Could you check a few things on this model? Use its own coordinates, in mm. Face numbers are marked on the shaded views. A direction names the side the tool comes from. Coordinates: 2 decimals unless noted, no trailing zeros. Loops run counter-clockwise (first coordinate to the right, second up) from the corner with the lowest first, then second, coordinate; pieces in that order, holes last. Notation, with made-up numbers: M -13,-6.75 L -8,-6.75 A22 cw -8,23.25 Z; hole C 86,26.25 d11. An arc over 180 degrees is marked long. Write each question's results on one line, items separated by ' | '.
```python
from build123d import *

# Parameters (mm, degrees)
SKETCH1_W                  = 26
SKETCH1_H                  = 24
BOSS_EXTRUDE1_DEPTH        = 12
CUT_EXTRUDE1_DEPTH         = 30.816103032
M3_CLEARANCE_HOLE1_D       = 3.242
M3_CLEARANCE_HOLE1_DEPTH   = 6.064115214
M3_CLEARANCE_HOLE1_TIP     = 0.935884786
F_4_5_4_5_DIAMETER_HOLE1_D = 4.5
CHAMFER1_SIZE              = 0.379


with BuildPart() as part:
    # Sketch1 → Boss-Extrude1 (new body)
    with BuildSketch(Plane.XY.offset(6)):
        with Locations((0, 12)):
            Rectangle(SKETCH1_W, SKETCH1_H)
    extrude(amount=-BOSS_EXTRUDE1_DEPTH)

    # Sketch2 → Cut-Extrude1 (cut, through all)
    with BuildSketch(Plane(origin=(0, 0, -6), x_dir=(-1, 0, 0), z_dir=(0, 0, -1))):
        with BuildLine():
            Line((3.01340754, 24), (-3.01340754, 24))
            ThreePointArc((-3.01340754, 24), (0, 21.825), (3.01340754, 24))
        make_face()
    extrude(amount=-CUT_EXTRUDE1_DEPTH, mode=Mode.SUBTRACT)

    # M3 Clearance Hole1
    with Locations(Plane(origin=(0, 24, 0), x_dir=(1, 0, 0), z_dir=(0, 1, 0))):
        with Locations((8, 0), (-8, 0)):
            Hole(M3_CLEARANCE_HOLE1_D / 2, depth=M3_CLEARANCE_HOLE1_DEPTH)
            with Locations((0, 0, -(M3_CLEARANCE_HOLE1_DEPTH + M3_CLEARANCE_HOLE1_TIP / 2))):  # 120° drill point
                Cone(0, M3_CLEARANCE_HOLE1_D / 2, M3_CLEARANCE_HOLE1_TIP, mode=Mode.SUBTRACT)

    # Ø4.5 (4.5) Diameter Hole1 (through all)
    with Locations(Plane.XY.offset(6)):
        with Locations((8, 5), (-8, 5)):
            Hole(F_4_5_4_5_DIAMETER_HOLE1_D / 2)

    # Chamfer1
    chamfer1_edges = [part.edges().sort_by_distance(p)[0] for p in [
        (-6.379, 24, 0),
        (9.621, 24, 0),
    ]]
    chamfer(chamfer1_edges, length=CHAMFER1_SIZE)


solid = part.part
```
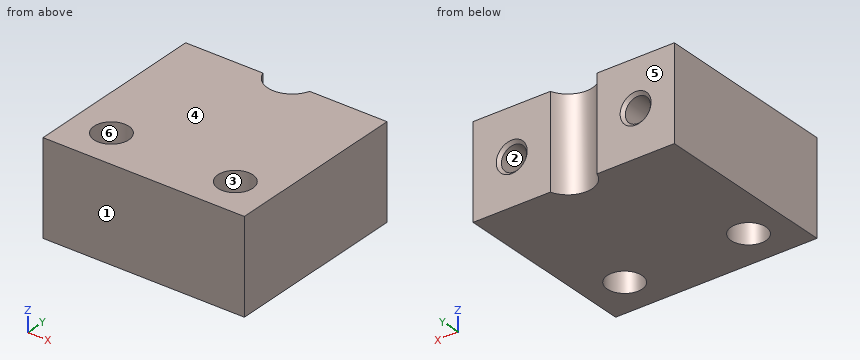
(1) Imagine slicing it at A-A, the plane y = 5. List the corners of the cut face in (x, z) for me.
Reported:
outline: M -13,-6 L -10.25,-6 L -10.25,6 L -13,6 Z; M -5.75,-6 L 5.75,-6 L 5.75,6 L -5.75,6 Z; M 10.25,-6 L 13,-6 L 13,6 L 10.25,6 Z
(2) Which directions (+Z, -Z, +X, -X, +Y, -Y) give clear straight access to the entire face, cutting with the end or side of a thin tool? Please do the marked faces 1 and 2.
Reported:
face 1: +Z, -Z, +X, -X, -Y | face 2: +Y
(3) Will this pin go through, and if not, where does the flat tip stop? P1, Ø3.5, axis at x = 8, y = 5, coming from the -Z side.
Reported:
P1: passes through
(4) Please list where these lines run through material, in increasing order: probe 1 along X at (y, z) = (19.7, 0); probe 2 along Y at (x, z) = (-8, 3.5); probe 3 along X at (y, z) = (5.5, 5.75). Write a range as from..to.
Reported:
probe 1: x = -13..-9.62, -6.38..6.38, 9.62..13 | probe 2: y = 0..2.75, 7.25..24 | probe 3: x = -13..-10.19, -5.81..5.81, 10.19..13
(5) Imagine slicing it at B-B, the plane z = -4.75. List the corners of the cut face in (x, y) for me (3 decimals).
Reported:
outline: M -13,0 L 13,0 L 13,24 L 3.013,24 A3.175 cw -3.013,24 L -13,24 Z; hole C -8,5 d4.5; hole C 8,5 d4.5
(6) If we mould it in two halves opening along Y, with no side actions, what happens to the marked faces 3, 4, 5 and 6? For each: released by +Y, released by -Y, zero draft, split by the parting line, or undercut.
Reported:
face 3: undercut | face 4: zero draft | face 5: released by +Y | face 6: undercut
(7) Imagine slicing it at C-C, the plane y = 21.5. List the corners of the cut face in (x, z) for me.
Reported:
outline: M -13,-6 L 13,-6 L 13,6 L -13,6 Z; hole C -8,0 d3.24; hole C 8,0 d3.24
